Study the drawing (mm; zero at the part's minimum x, y, z) and answer. Round coordinates to 2 decimals unless told otherwise and drop trailing zeros. Order: outer loops, then holes, each group sorted by start corner. A loop starts at its lowest first (then second) coordinate and runs counter-clockwise, first axis right, second up. Notation, with made-up numbers: M 41,29.25 L 51,29.25 A32 ccw 51,67.25 Z; hole C 77,80 d6. An arc over 180 degrees is marked long. Put each result on its own line as item: value. Start each with the question number.
1. The part is cut by section A-A (z = 85.99). Give the vertices of the cut face in (x, y) (3 decimals).
2. Consider line 1 (X direction, y = 2.25, z = 73); line 2 (Z direction, x = 77, y = 0.25); line 3 (Z direction, x = 26, y = 2.1) (1 decimal). Determine where each line is inside the solid, lowest interval first.
3. The part is cut by section C-C (x = 85.99). Give the vertices of the cut face in (y, z) (3 decimals).
4. The part is cut by section D-D (x = 52.5). Give the vertices of the cut face in (y, z) (1 decimal).
5. Each of these flat-tipped pins is pushed along its axis until it touches: pin 1 Ø1 at (x, z) = (91.5, 74.5) entering from -Y; pin 2 Ø1 at (x, y) = (126, 0.5) entering from +Z; pin 3 Ø4 at (x, z) = (74.676, 85.99) entering from -Y. Where does it stop, or does it pass through?
6. The part is cut by section B-B (y = 0.55). Count the separate pieces of the cut face and the enclosed holes in it, then the cut area to 3 significant figures.
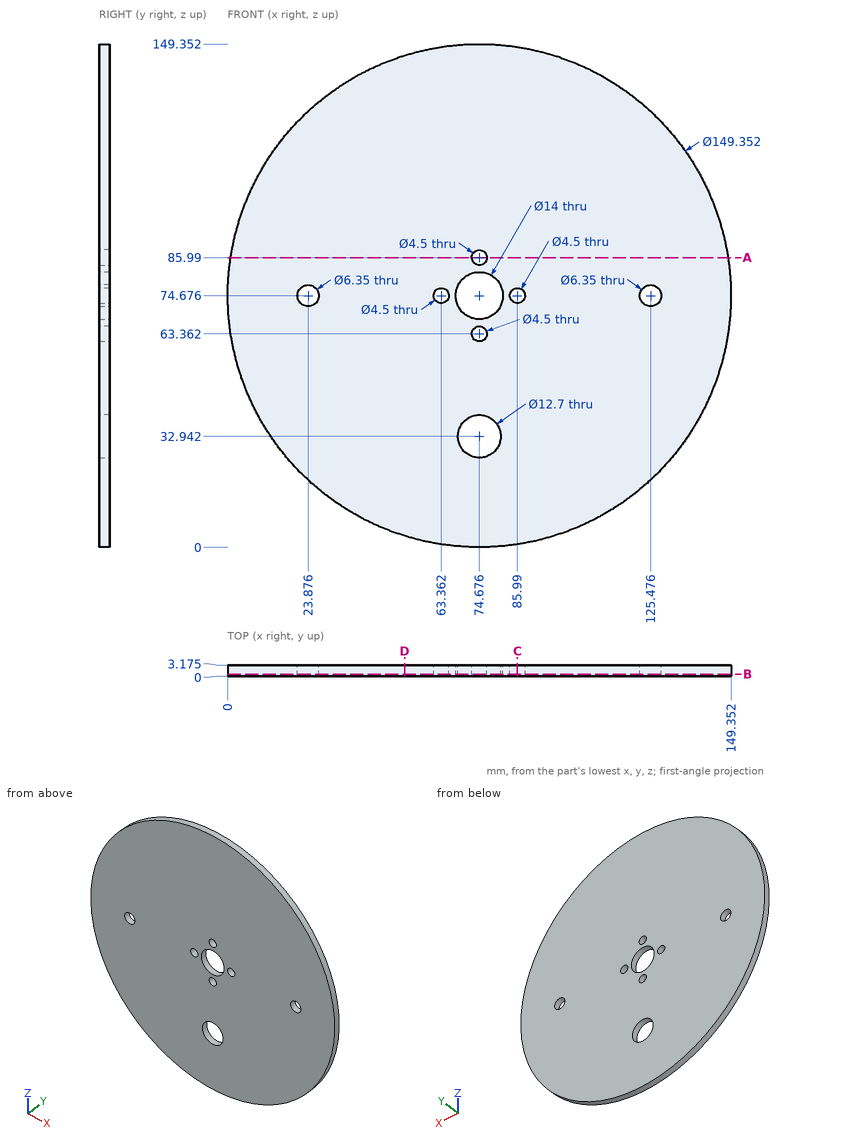
Resolved:
1. outline: M 0.862,0 L 72.426,0 L 72.426,3.175 L 0.862,3.175 Z; M 76.926,0 L 148.49,0 L 148.49,3.175 L 76.926,3.175 Z
2. line 1: 0.02 to 21.18, 26.57 to 61.86, 64.86 to 67.88, 81.47 to 84.49, 87.49 to 122.78, 128.17 to 149.33
2. line 2: 0.04 to 27.03, 38.85 to 68.07, 81.28 to 149.32
2. line 3: 18 to 72.3, 77 to 131.3
3. outline: M 0,0.862 L 3.175,0.862 L 3.175,72.426 L 0,72.426 Z; M 0,76.926 L 3.175,76.926 L 3.175,148.49 L 0,148.49 Z
4. outline: M 0,3.4 L 3.2,3.4 L 3.2,146 L 0,146 Z
5. pin 1: y = 0
5. pin 2: z = 129.39
5. pin 3: through
6. separate pieces: 1
6. enclosed holes: 8
6. area: 17,100 mm2
